Autodesk Inventor part; units mm, degrees
ref_plane "YZ Plane" through (0, 0, 0) normal (1, 0, 0) x (0, 1, 0)
ref_plane "XZ Plane" through (0, 0, 0) normal (0, 1, 0) x (-1, 0, 0)
ref_plane "XY Plane" through (0, 0, 0) normal (0, 0, 1) x (1, 0, 0)
sketch "Skizze1" plane through (0, 0, 0) normal (0, 0, 1) x (1, 0, 0)
  line L0 (-11.356, -4.7452) -> (20.644, -4.7452)
  line L1 (20.644, -4.7452) -> (20.644, 5.7548)
  line L2 (20.644, 5.7548) -> (-11.356, 5.7548)
  line L3 (-11.356, 5.7548) -> (-11.356, -4.7452)
  point P0 (0, 0)
  dimension "d0" = 32
  dimension "d1" = 10.5
extrude "Extrusion1" add sketch "Skizze1" along normal blind 9
sketch "Skizze2" plane through (0, 0, 9) normal (0, 0, 1) x (1, 0, 0)
  line L0 (20.644, -4.7452) -> (20.644, 5.7548)
  line L1 (-11.356, -4.7452) -> (20.644, -4.7452)
  point P0 (0, 0)
  point P1 (-3.86, -0.9952)
  point P2 (4.644, -0.9952)
  point P3 (13.148, -0.9952)
  dimension "d4" = 8.504
  dimension "d5" = 8.504
  dimension "d6" = 7.496
  dimension "d20" = 3.75
  dimension "d21" = 3.75
hole "Bohrung1" at (-3.86, -0.9952, 9) at (4.644, -0.9952, 9) at (13.148, -0.9952, 9) direction (0, 0, -1) diameter 5.15 end through all
sketch "Skizze3" plane through (0, 0, 9) normal (0, 0, 1) x (1, 0, 0)
  point P0 (0, 0)
sketch "Skizze4" plane through (-11.356, -4.7452, 0) normal (0, -1, 0) x (1, 0, 0)
  line L0 (11.575, 6.55) -> (20.425, 6.55)
  line L1 (20.425, 6.55) -> (20.425, 2.45)
  line L2 (20.425, 2.45) -> (11.575, 2.45)
  line L3 (11.575, 2.45) -> (11.575, 6.55)
  line L4 (32, 0) -> (32, 9)
  line L5 (0, 9) -> (32, 9)
  point P0 (11.356, 0)
  dimension "d14" = 8.85
  dimension "d15" = 4.1
  dimension "d16" = 11.575
  dimension "d17" = 2.45
extrude "Extrusion2" cut sketch "Skizze4" against normal blind 9.3
sketch "Skizze5" plane through (0, 0, 9) normal (0, 0, 1) x (1, 0, 0)
  point P0 (0, 0)
sketch "Skizze6" plane through (-11.356, -4.7452, 0) normal (0, -1, 0) x (1, 0, 0)
  line L0 (4.905, 0) -> (9.905, 0)
  line L1 (9.905, 0) -> (9.905, 2)
  line L2 (9.905, 2) -> (4.905, 2)
  line L3 (4.905, 2) -> (4.905, 0)
  line L4 (0, 0) -> (0, 9)
  point P0 (11.356, 0)
  dimension "d22" = 5
  dimension "d23" = 2
  dimension "d24" = 4.905
sketch "Skizze7" plane through (-11.356, -4.7452, 0) normal (0, -1, 0) x (1, 0, 0)
  point P0 (11.356, 0)
extrude "Extrusion3" add sketch "Skizze6" along normal blind 5
sketch "Skizze8" plane through (-6.451, -4.7452, 2) normal (0, 0, 1) x (1, 0, 0)
  line L0 (0, -5) -> (5, -5)
  line L1 (0, 0) -> (0, -5)
  line L2 (5, -5) -> (0, -5)
  line L3 (0, -5) -> (0, 0)
  line L4 (0, 0) -> (5, 0)
  line L5 (5, 0) -> (5, -5)
  point P0 (6.451, 4.7452)
extrude "Extrusion4" add sketch "Skizze8" along normal blind 22
sketch "Skizze9" plane through (-6.451, -4.7452, 24) normal (0, 0, 1) x (1, 0, 0)
  line L0 (0, -5) -> (5, -5)
  line L1 (1.875, -5) -> (3.125, -5)
  line L2 (3.125, -5) -> (3.125, -0.952)
  line L3 (3.125, -0.952) -> (1.875, -0.952)
  line L4 (1.875, -0.952) -> (1.875, -5)
  line L5 (5, -5) -> (5, 0)
  line L6 (0, 0) -> (0, -5)
  point P0 (6.451, 4.7452)
  dimension "d29" = 1.875
  dimension "d30" = 1.875
  dimension "d31" = 4.048
extrude "Extrusion5" cut sketch "Skizze9" against normal blind 22
properties part number "Objektträgerhalter 3b Neu"
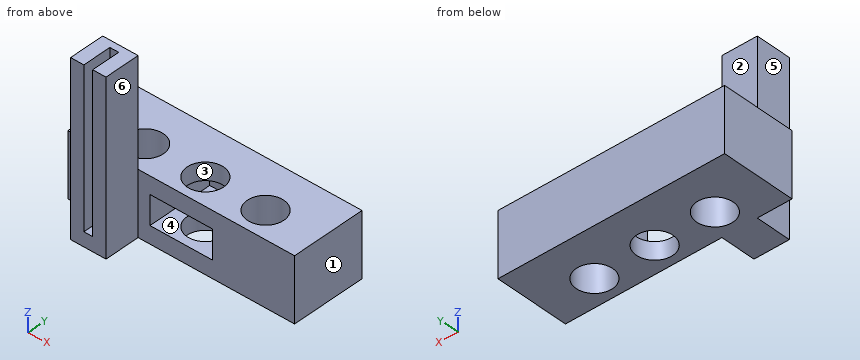
The listing builds one solid part. Answer for the finished solid, in the listing's coordinates (mm). Face numbers are marked on the shaded views. A direction names the side the tool comes from. Give positions to 0.01 mm unless a question says otherwise; leave off trailing zeros. Order: outer loops, then holes, each group sorted by start corner. A loop starts at its lowest first (then second) coordinate and runs counter-clockwise, first axis right, second up. Notation, with made-up numbers: (51, 57.5) -> (90, 57.5) arc R21 ccw to (90, 76.5) -> close; hole circle Ø4 at (-3, 34). An arc over 180 degrees is marked (long way). One line per item, written item: value.
1) Find the intervals of material crossed by line 1 (Z direction, x = 3.5, y = 2.5); line 2 (X direction, y = -8, z = 19.25); line 3 (Y direction, x = -3.86, z = 6.5), in increasing order.
Reported:
line 1: z = 0 to 2.45, 6.55 to 9
line 2: x = -6.45 to -4.58, -3.33 to -1.45
line 3: y = -5.7 to -3.57, 1.58 to 5.75
2) A tool of negligible diameter and unlimited length cuts with its end or side. For the marked faces 4, 5 and 6, from which of +Z, -Z, +X, -X, +Y, -Y can it reach the whole face along a straight path? Write none if from no direction.
Reported:
face 4: -Y
face 5: +Z, -Z, -X, -Y
face 6: +Z, -Z, +X, -Y
3) Find section D-D, the plane z = 5. Determine the outline of the cut face in (x, y) (3 decimals).
Reported:
outline: (-11.356, -4.745) -> (-6.451, -4.745) -> (-6.451, -9.745) -> (-4.576, -9.745) -> (-4.576, -5.697) -> (-3.326, -5.697) -> (-3.326, -9.745) -> (-1.451, -9.745) -> (-1.451, -4.745) -> (0.219, -4.745) -> (0.219, 4.555) -> (9.069, 4.555) -> (9.069, -4.745) -> (20.644, -4.745) -> (20.644, 5.755) -> (-11.356, 5.755) -> close; hole circle Ø5.15 at (-3.86, -0.995); hole circle Ø5.15 at (13.148, -0.995)
4) Find section A-A, the plane x = -3.86. Determine the outline of the cut face in (y, z).
Reported:
outline: (-9.75, 0) -> (-3.57, 0) -> (-3.57, 9) -> (-4.75, 9) -> (-4.75, 24) -> (-5.7, 24) -> (-5.7, 2) -> (-9.75, 2) -> close; (1.58, 0) -> (5.75, 0) -> (5.75, 9) -> (1.58, 9) -> close
5) Flat-ended cylindrical pins translate along their axes: P1, Ø2, axis at y = -8, z = 8.5, coming from the -X side; P2, Ø4, axis at x = -5, z = 13, coming from the +Y side; P3, Ø0.6, axis at x = -4, y = -8, coming from the +Z side; P4, Ø5, axis at x = -0.5, y = -7, coming from the -Z side. Find the tip coordinate at first contact, or state that the pin passes through.
Reported:
P1: stops at x = -6.45
P2: stops at y = -4.75
P3: stops at z = 2
P4: stops at z = 0
6) Find section C-C, the plane z = 14. Determine the outline of the cut face in (x, y), plus the area to 3 significant figures.
Reported:
outline: (-6.45, -9.75) -> (-4.58, -9.75) -> (-4.58, -5.7) -> (-3.33, -5.7) -> (-3.33, -9.75) -> (-1.45, -9.75) -> (-1.45, -4.75) -> (-6.45, -4.75) -> close
area: 19.9 mm^2
7) Find section B-B, the plane y = 0. Determine the outline of the cut face in (x, z).
Reported:
outline: (-11.36, 0) -> (-6.23, 0) -> (-6.23, 9) -> (-11.36, 9) -> close; (-1.49, 0) -> (2.27, 0) -> (2.27, 2.45) -> (0.22, 2.45) -> (0.22, 6.55) -> (2.27, 6.55) -> (2.27, 9) -> (-1.49, 9) -> close; (7.02, 0) -> (10.77, 0) -> (10.77, 9) -> (7.02, 9) -> (7.02, 6.55) -> (9.07, 6.55) -> (9.07, 2.45) -> (7.02, 2.45) -> close; (15.52, 0) -> (20.64, 0) -> (20.64, 9) -> (15.52, 9) -> close
8) Determine the mould class of the marked faces 1, 2 and 3 for opening direction Y: pulls with the +Y half, pulls with the -Y half, needs draft (parallel to the pull), parting line crosses it, or undercut.
Reported:
face 1: needs draft
face 2: pulls with the +Y half
face 3: undercut
